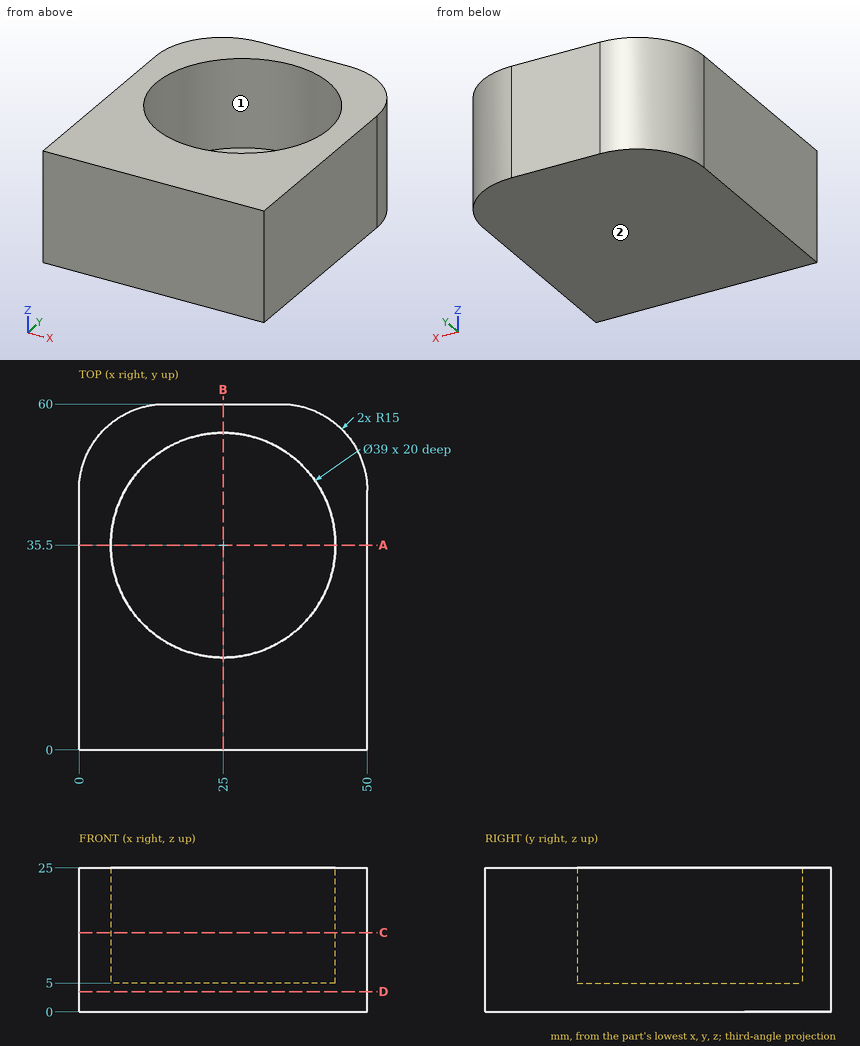
Job drawing, mm, ordinate dimensions from the low corner. One solid piece. A direction names the side the tool comes from. Round coordinates to 2 decimals unless told otherwise and drop trailing zeros. Write each loop counter-clockwise with the first axis right and the second up, starting at its lowest first coordinate (ties: lowest second). Pieces come first, ordered by that corner, then holes.
1) Band-saw the part on C-C, the plane z = 13.75. List the corners of the cut face in (x, y).
2) Band-saw the part on D-D, the plane z = 3.5. List the corners of the cut face in (x, y).
3) Drill centre lines: probe 1 along Y at (x, z) = (25, 11.75); probe 2 along X at (y, z) = (35.5, 17); probe 3 along Z at (x, y) = (6.5, 30.5). Where is each one in solid material? Low to high.
4) Band-saw the part on A-A, the plane y = 35.5. List the corners of the cut face in (x, z).
5) 3-axis set-ups, long thin cutter, end or side, ignore diameter. For the marked faces 1 and 2: which of +Z, -Z, +X, -X, +Y, -Y reach the whole face in a straight line?
6) Band-saw the part on B-B, the plane x = 25. List the corners of the cut face in (y, z).
7) Pin check, flat tips, straight feed: pin 1 (12 mm diameter, centred on x = 21.5, y = 29.5, fed in from -Z); pin 2 (19.5 mm diameter, centred on x = 26.5, y = 34, fed in from +Z); pin 3 (1 mm diameter, centred on y = 54, z = 4.5, fed in from +X); pin 4 (1 mm diameter, centred on y = 49, z = 16.5, fed in from -X). Stop position of each tip, or through.
Ans:
1. outline: (0, 0) - (50, 0) - (50, 45) arc R15 ccw to (35, 60) - (15, 60) arc R15 ccw to (0, 45) - close; hole circle Ø39 at (25, 35.5)
2. outline: (0, 0) - (50, 0) - (50, 45) arc R15 ccw to (35, 60) - (15, 60) arc R15 ccw to (0, 45) - close
3. probe 1: y = 0 to 16, 55 to 60
3. probe 2: x = 0 to 5.5, 44.5 to 50
3. probe 3: z = 0 to 5
4. outline: (0, 0) - (50, 0) - (50, 25) - (44.5, 25) - (44.5, 5) - (5.5, 5) - (5.5, 25) - (0, 25) - close
5. face 1: +Z
5. face 2: -Z, +X, -X, +Y, -Y
6. outline: (0, 0) - (60, 0) - (60, 25) - (55, 25) - (55, 5) - (16, 5) - (16, 25) - (0, 25) - close
7. pin 1: stops at z = 0
7. pin 2: stops at z = 5
7. pin 3: stops at x = 47.36
7. pin 4: stops at x = 0.41
